from build123d import *
from build123d.topology import SkipClean

# Parameters (mm, degrees)
ESQUISSE1_R                = 30
BOSS_EXTRU_1_DEPTH         = 30
ESQUISSE2_R                = 35
BOSS_EXTRU_2_DEPTH         = 10
CHANFREIN1_SIZE            = 5
ESQUISSE3_R                = 5.5
ENL_V_MAT_EXTRU_1_DEPTH    = 40
BOSS_EXTRU_6_DEPTH         = 10
ESQUISSE5_R                = 2.25
R_P_TITION_LIN_AIRE1_COUNT = 2
R_P_TITION_LIN_AIRE1_PITCH = 10


with BuildPart() as part:
    # Esquisse1 → Boss.-Extru.1 (new body)
    with BuildSketch(Plane.XY):
        Circle(ESQUISSE1_R)
    extrude(amount=BOSS_EXTRU_1_DEPTH)

    # Esquisse2 → Boss.-Extru.2 (add)
    with BuildSketch(Plane(origin=(0, 0, 0), x_dir=(-1, 0, 0), z_dir=(0, 0, -1))):
        Circle(ESQUISSE2_R)
    extrude(amount=BOSS_EXTRU_2_DEPTH)

    # Chanfrein1
    chanfrein1_edges = [part.edges().sort_by_distance(p)[0] for p in [
        (-30, 0, 30),
    ]]
    chamfer(chanfrein1_edges, length=CHANFREIN1_SIZE)

    # Esquisse3 → Enlèv. mat.-Extru.1 (cut)
    with BuildSketch(Plane(origin=(0, 0, -10), x_dir=(-1, 0, 0), z_dir=(0, 0, -1))):
        Circle(ESQUISSE3_R)
    extrude(amount=-ENL_V_MAT_EXTRU_1_DEPTH, mode=Mode.SUBTRACT)

    # Esquisse4 → Boss.-Extru.6 (add)
    with SkipClean():  # the faces are left unmerged after this step: merging them gives an invalid solid
        with BuildSketch(Plane.XY.offset(30)):
            with BuildLine():
                Line((0, 10), (0, 5.5))
                ThreePointArc((0, 5.5), (-5.5, 0), (0, -5.5))
                Line((0, -5.5), (0, -10))
                Line((0, -10), (-2.5, -10))
                Line((-2.5, -10), (-3.5, -10))
                Line((-3.5, -10), (-6.284490288, -10))
                Line((-6.284490288, -10), (-6.284490288, 10))
                Line((-6.284490288, 10), (-3.5, 10))
                Line((-3.5, 10), (-2.5, 10))
                Line((-2.5, 10), (0, 10))
            make_face()
        extrude(amount=BOSS_EXTRU_6_DEPTH)
    add(part.part.scale(1), mode=Mode.REPLACE)  # the faces are merged on a copy

    # Enlèvement de matière-Balayage1: sweep along a path in Esquisse6
    with BuildLine(Plane.XY.offset(8)) as enl_vement_de_mati_re_balayage1_path:
        CenterArc((0, 0), 23.00163751, 0, 360)
    # Esquisse5 → Enlèvement de matière-Balayage1 (sweep, cut)
    with BuildSketch(Plane(origin=(0, 0, 0), x_dir=(0, 0, -1), z_dir=(1, 0, 0))):
        with Locations((-7.687500001, -30)):
            Circle(ESQUISSE5_R)
    enl_vement_de_mati_re_balayage1 = sweep(path=enl_vement_de_mati_re_balayage1_path.line, mode=Mode.SUBTRACT)

    # Répétition linéaire1: Enlèvement de matière-Balayage1 ×2
    with Locations(*[(0, 0, i * R_P_TITION_LIN_AIRE1_PITCH) for i in range(1, R_P_TITION_LIN_AIRE1_COUNT)]):
        add(enl_vement_de_mati_re_balayage1, mode=Mode.SUBTRACT)


solid = part.part
Design review of the part built by this model. Coordinates are the model's own, in mm. A direction names the side the tool comes from. Give positions to 0.01 mm unless a question says otherwise; leave off trailing zeros. Order: outer loops, then holes, each group sorted by start corner. A loop starts at its lowest first (then second) coordinate and runs counter-clockwise, first axis right, second up. Notation, with made-up numbers: (28, -9) - (42, -9) arc R21 ccw to (42, 5) - close; hole circle Ø11 at (72, 87). An arc over 180 degrees is marked (long way). Use CSV: the item, a comma, the result in double quotes. Start each with the question number.
Q1. For P1, Ø1, axis at x = 4, z = 17, coming from the -Y side; P2, Ø1.3, axis at y = -8.5, z = 34, coming from the +X side; P3, Ø8, axis at x = -16, z = 14, coming from the -Y side, all flat-tipped, find the tip position at first contact; note any pin that passes through.
Q2. For line 1 (Y direction, x = 0, z = 21); line 2 (Z direction, x = -6.5, y = 29); line 3 (Z direction, x = -23.5, y = 16.5), list the stretches that pass through material, from the lowest coordinate up.
Q3. Machinability: for faces 1 (the face through (-29.97, 1.32, 22.43)), 2 (the face through (-3, 10, 35)), 3 (the face through (0, -8, 35)), 4 (the face through (-3, -10, 35)), which of the approach directions +Z, -Z, +X, -X, +Y, -Y give a long, thin tool a straight path to every point of the face, cutting with its end or side? Answer none if there is none.
Q4. Take a section at B-B (z = 4). State the section outline as (x, y) points.
Q5. Take a section at C-C (z = -4.5). State the section outline as (x, y) points.
Q6. Take a section at A-A (y = 0). State the section outline as (x, z) points.
Calculated:
1,P1,"stops at y = -27.81"
1,P2,"stops at x = 0"
1,P3,"stops at y = -27.5"
2,line 1,"y = -30 to -5.5, 5.5 to 30"
2,line 2,"z = -10 to 5.46, 9.92 to 15.46, 19.92 to 25.28"
2,line 3,"z = -10 to 5.84, 9.53 to 15.84, 19.53 to 26.29"
3,face 1,"+Z"
3,face 2,"+Z, +X, -X, +Y"
3,face 3,"+Z, +X, +Y, -Y"
3,face 4,"+Z, +X, -X, -Y"
4,outline,"circle Ø60 at (0, 0); hole circle Ø11 at (0, 0)"
5,outline,"circle Ø70 at (0, 0); hole circle Ø11 at (0, 0)"
6,outline,"(-35, -10) - (-5.5, -10) - (-5.5, 40) - (-6.28, 40) - (-6.28, 30) - (-25, 30) - (-30, 25) - (-30, 19.94) arc R2.25 cw to (-30, 15.44) - (-30, 9.94) arc R2.25 cw to (-30, 5.44) - (-30, 0) - (-35, 0) - close; (5.5, -10) - (35, -10) - (35, 0) - (30, 0) - (30, 5.44) arc R2.25 cw to (30, 9.94) - (30, 15.44) arc R2.25 cw to (30, 19.94) - (30, 25) - (25, 30) - (5.5, 30) - close"
